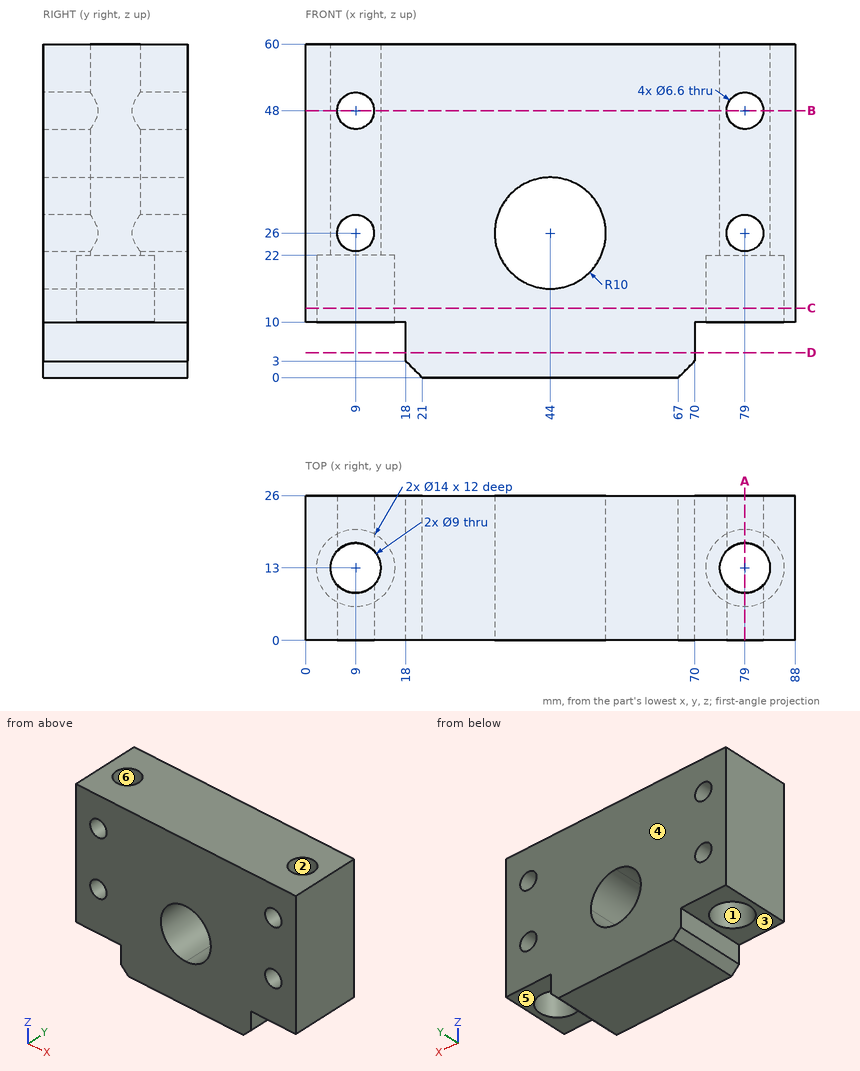
Study the drawing (mm; zero at the part's minimum x, y, z) and answer. A direction names the side the tool comes from. Give positions to 0.01 mm unless a question says otherwise; leave off trailing zeros. Write each loop counter-clockwise with the first axis right and the second up, starting at its lowest first coordinate (ties: lowest second). Pieces come first, ordered by that corner, then holes. Notation, with made-up numbers: (61.5, 61) - (117.5, 61) arc R21 cw to (117.5, 76) - close; hole circle Ø6 at (89, 63.5). An arc over 180 degrees is marked (long way). Use a Markdown table: item, result.
1. Each of these flat-tipped pins is pushed along its axis until it touches: P1, Ø10.5, axis at x = 79, y = 13, coming from the -Z side; P2, Ø2, axis at y = 19, z = 6, coming from the -X side; P3, Ø3.5, axis at y = 18.5, z = 5, coming from the +X side. Where does it stop, or does it pass through?
Values follow:
| item | result |
|---|---|
| P1 | stops at z = 22 |
| P2 | stops at x = 18 |
| P3 | stops at x = 70 |
2. Section A-A on x = 79 is taken. Write down the section's boundary in (y, z).
Values follow:
| item | result |
|---|---|
| outline | (0, 10) - (6, 10) - (6, 22) - (8.5, 22) - (8.5, 22.7) - (0, 22.7) - close; (0, 29.3) - (8.5, 29.3) - (8.5, 44.7) - (0, 44.7) - close; (0, 51.3) - (8.5, 51.3) - (8.5, 60) - (0, 60) - close; (17.5, 22) - (20, 22) - (20, 10) - (26, 10) - (26, 22.7) - (17.5, 22.7) - close; (17.5, 29.3) - (26, 29.3) - (26, 44.7) - (17.5, 44.7) - close; (17.5, 51.3) - (26, 51.3) - (26, 60) - (17.5, 60) - close |
3. Section B-B on z = 48 is taken. Write down the section's boundary in (x, y), plus the area to 3 significant figures.
Values follow:
| item | result |
|---|---|
| outline | (0, 0) - (5.7, 0) - (5.7, 9.94) arc R4.5 cw to (5.7, 16.06) - (5.7, 26) - (0, 26) - close; (12.3, 0) - (75.7, 0) - (75.7, 9.94) arc R4.5 cw to (75.7, 16.06) - (75.7, 26) - (12.3, 26) - (12.3, 16.06) arc R4.5 cw to (12.3, 9.94) - close; (82.3, 0) - (88, 0) - (88, 26) - (82.3, 26) - (82.3, 16.06) arc R4.5 cw to (82.3, 9.94) - close |
| area | 1,920 mm² |
4. A tool of negligible diameter and unlimited length cuts with its end or side. For the marked faces 1, 2 and 3, from which of +Z, -Z, +X, -X, +Y, -Y can it reach the whole face along a straight path? Write none if from no direction.
Values follow:
| item | result |
|---|---|
| face 1 | -Z |
| face 2 | +Z, -Z |
| face 3 | -Z, -X, +Y, -Y |
5. For a pull along Y with two mould halves and no side action, classify the marked faces 4, 5 and 6 as released by +Y, released by -Y, zero draft, split by the parting line, or undercut.
Values follow:
| item | result |
|---|---|
| face 4 | released by +Y |
| face 5 | zero draft |
| face 6 | undercut |
6. Section C-C on z = 12.5 is taken. Write down the section's boundary in (x, y), plus the area to 3 significant figures.
Values follow:
| item | result |
|---|---|
| outline | (0, 0) - (88, 0) - (88, 26) - (0, 26) - close; hole circle Ø14 at (9, 13); hole circle Ø14 at (79, 13) |
| area | 1,980 mm² |
7. Section D-D on z = 4.5 is taken. Write down the section's boundary in (x, y), plus the area to 3 significant figures.
Values follow:
| item | result |
|---|---|
| outline | (18, 0) - (70, 0) - (70, 26) - (18, 26) - close |
| area | 1,350 mm² |
8. Find the intervals of material crossed by probe 1 along X at (y, z) = (20.5, 26); probe 2 along Z at (x, y) = (79, 22.75); probe 3 along X at (y, z) = (12.5, 18), in increasing order. Write a range as from..to.
Values follow:
| item | result |
|---|---|
| probe 1 | x = 0..5.7, 12.3..34, 54..75.7, 82.3..88 |
| probe 2 | z = 10..22.7, 29.3..44.7, 51.3..60 |
| probe 3 | x = 0..2.02, 15.98..38, 50..72.02, 85.98..88 |
